Geometry: final body of the model. Coordinates: model frame, mm. Face numbers are marked on the shaded views. A direction names the side the tool comes from. Coordinates: 2 decimals unless noted, no trailing zeros. Loops run counter-clockwise (first coordinate to the right, second up) from the corner with the lowest first, then second, coordinate; pieces in that order, holes last. Notation, with made-up numbers: (-35.5, 42) - (-6.5, 42) arc R11 ccw to (-6.5, 62) - close; hole circle Ø9 at (66, 21). An arc over 180 degrees is marked (long way). Return JSON: item names as keys, results as strings.
from build123d import *

# Parameters (mm, degrees)
SKETCH1_W          = 50.8
SKETCH1_H          = 28.575
EXTRUDE1_DEPTH     = 46.7868
LPATTERN1_COUNT    = 2
LPATTERN1_PITCH    = 27.94
SKETCH5_R          = 13.5001
EXTRUDE2_DEPTH     = 5.969
SKETCH6_W          = 6.3373
SKETCH6_H          = 10.541
CUT_EXTRUDE4_DEPTH = 30.48
HOLE1_D            = 7.137
HOLE1_DEPTH        = 46.7868
HOLE2_D            = 7.137
HOLE2_DEPTH        = 28.575


with BuildPart() as part:
    # Sketch1 → Extrude1 (new body)
    with BuildSketch(Plane(origin=(0, 0, 0), x_dir=(0, 0, -1), z_dir=(1, 0, 0))):
        with Locations((2.3876, 0)):
            Rectangle(SKETCH1_W, SKETCH1_H)
    extrude(amount=EXTRUDE1_DEPTH)

    # S2D0002 → Cut-Revolve1 (revolve, cut)
    with BuildSketch(Plane(origin=(0, 4.7625, 0), x_dir=(-1, 0, 0), z_dir=(0, 1, 0)), mode=Mode.PRIVATE) as cut_revolve1_sk:
        Polygon((-14.5415, -27.5336), (-18.161, -27.5336), (-18.161, -27.7876), (-9.525, -27.7876), (-9.525, -14.0716), (-13.9446, -14.0716), (-13.9446, -26.9113), (-14.5415, -27.5082), align=None)
    cut_revolve1 = revolve(cut_revolve1_sk.sketch.rotate(Axis((9.525, 4.7625, -19.13842003), (0, 0, 1)), 180), axis=Axis((9.525, 4.7625, -19.13842003), (0, 0, 1)), mode=Mode.SUBTRACT)  # turned: the seam where the file's is

    # LPattern1: Cut-Revolve1 ×2
    with Locations(*[(i * LPATTERN1_PITCH, 0, 0) for i in range(1, LPATTERN1_COUNT)]):
        add(cut_revolve1, mode=Mode.SUBTRACT)

    # Sketch5 → Extrude2 (add)
    with BuildSketch(Plane.ZY):
        Circle(SKETCH5_R)
    extrude(amount=EXTRUDE2_DEPTH)

    # Sketch6 → Revolve1 (revolve)
    with BuildSketch(Plane(origin=(0, 0, 0), x_dir=(0, 0, 1), z_dir=(0, -1, 0)), mode=Mode.PRIVATE) as revolve1_sk:
        with Locations((-3.16865, 11.2395)):
            Rectangle(SKETCH6_W, SKETCH6_H)
    revolve(revolve1_sk.sketch.rotate(Axis((5.754582971, 0, 0), (-1, 0, 0)), 180), axis=Axis((5.754582971, 0, 0), (-1, 0, 0)))  # turned: the seam where the file's is

    # S2D0001 → Cut-Revolve4 (revolve, cut)
    with BuildSketch(Plane(origin=(-18.511260017, 3.2639, 0), x_dir=(0, 1, 0), z_dir=(0, 0, 1)), mode=Mode.PRIVATE) as cut_revolve4_sk:
        Polygon((-0.7493, -3.365076823), (-0.7493, -18.003260017), (-3.2639, -19.51418413), (-3.2639, -2.001260017), (0.0381, -2.001260017), align=None)
    revolve(cut_revolve4_sk.sketch.rotate(Axis((0, 0, 0), (-1, 0, 0)), 90), axis=Axis((0, 0, 0), (-1, 0, 0)), mode=Mode.SUBTRACT)  # turned: the seam where the file's is

    # Sketch8 → Cut-Revolve5 (revolve, cut)
    with BuildSketch(Plane(origin=(0, 0, 0), x_dir=(0, 0, -1), z_dir=(0, 1, 0)), mode=Mode.PRIVATE) as cut_revolve5_sk:
        with BuildLine():
            Line((-6.3373, 10.1854), (-6.096, 10.9474))
            Line((-6.096, 10.9474), (-6.096, 15.494))
            ThreePointArc((-6.096, 15.494), (-5.995678675, 16.037796865), (-5.707922533, 16.51))
            Line((-5.707922533, 16.51), (-6.3373, 16.51))
            Line((-6.3373, 16.51), (-6.3373, 10.1854))
        make_face()
    revolve(cut_revolve5_sk.sketch.rotate(Axis((-12.65936, 0, 0), (-1, 0, 0)), 180), axis=Axis((-12.65936, 0, 0), (-1, 0, 0)), mode=Mode.SUBTRACT)  # turned: the seam where the file's is

    # Sketch12 → Cut-Extrude4 (cut, symmetric)
    with BuildSketch(Plane(origin=(0, 0, 0), x_dir=(0, -1, 0), z_dir=(0, 0, -1))):
        Polygon((5.461, 16.51), (5.461, 11.7348), (6.096, 11.0998), (6.096, 16.51), align=None)
        Polygon((-5.461, 16.51), (-5.461, 11.7348), (-6.096, 11.0998), (-6.096, 16.51), align=None)
    extrude(amount=CUT_EXTRUDE4_DEPTH, both=True, mode=Mode.SUBTRACT)

    # Hole1
    with Locations(Plane.ZY):
        with Locations((-16.6878, -7.9248), (16.6624, 7.9502)):
            Hole(HOLE1_D / 2, depth=HOLE1_DEPTH)

    # Hole2
    with Locations(Plane(origin=(0, 14.2875, 0), x_dir=(-1, 0, 0), z_dir=(0, 1, 0))):
        with Locations((-23.3172, -16.6878), (-23.3172, 16.6624)):
            Hole(HOLE2_D / 2, depth=HOLE2_DEPTH)


solid = part.part
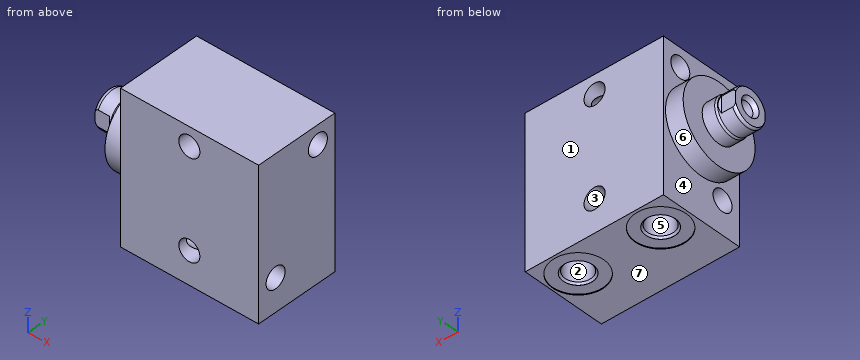
Item 1: Section query C-C, the plane y = -1.75. Count the separate pieces of the cut face and the enclosed holes in it, and give its area (3 significant figures).
Worked out:
{"separate pieces": "1", "enclosed holes": "2", "area": "2,520 mm^2"}
Item 2: Ray query, probe 1 along X at (y, z) = (8, -22.5); probe 2 along Z at (x, y) = (26, 5.5); probe 3 along X at (y, z) = (7.25, 6). Return the intervals inside material, ascending. Write a range as from..to.
Worked out:
{"probe 1": "0..6.52, 12.53..34.46, 40.47..46.79", "probe 2": "-27.79..-19.04, -14.33..14.07, 19.26..23.01", "probe 3": "-5.97..46.79"}
Item 3: Mould query, pull axis X, two halves, no side actions, for the marked faces 1, 2, 3 and 4. Classes: +X half, -X half, draft (parallel to the pull), parting line (faces both ways), or undercut.
Worked out:
{"face 1": "draft", "face 2": "undercut", "face 3": "undercut", "face 4": "-X half"}
Item 4: Reachability of the marked faces 5, 6 and 7 from +Z, -Z, +X, -X, +Y, -Y: full face, straight path, thin tool, end or side. Return the list, or none.
Worked out:
{"face 5": "-Z", "face 6": "-X", "face 7": "-Z, +X, -X, +Y, -Y"}
Item 5: First-contact query: pin 1 Ø11.5 at (y, z) = (7.95, 16.66) entering from -X; pin 2 Ø4 at (x, z) = (-14.5, -1) entering from -Y; pin 3 Ø8 at (x, y) = (37.47, 4.76) entering from -Z. Flat tips, straight axial feed; report the tip coordinate or a pass-through.
Worked out:
{"pin 1": "x = -5.97", "pin 2": "y = -5.46", "pin 3": "z = -14.07"}
Item 6: Section query A-A, the plane z = -19. Return loops of the section in (x, y) (1 decimal).
Worked out:
{"outline": "(0, -14.3) - (20.6, -14.3) - (20.6, -10.6) - (0, -10.6) - close; (0, -5.2) - (20.6, -5.2) - (20.6, 14.3) - (0, 14.3) - close; (26, -14.3) - (46.8, -14.3) - (46.8, -10.6) - (26, -10.6) - close; (26, -5.2) - (46.8, -5.2) - (46.8, 14.3) - (26, 14.3) - close; hole circle Ø8.8 at (9.5, 4.8); hole circle Ø8.8 at (37.5, 4.8)"}
Item 7: Section query B-B, the plane z = 17.5. Return loops of the section in (x, y), and give its area (3 significant figures).
Worked out:
{"outline": "(0, -14.29) - (19.85, -14.29) - (19.85, 4.48) - (0, 4.48) - close; (0, 11.42) - (19.85, 11.42) - (19.85, 14.29) - (0, 14.29) - close; (26.79, -14.29) - (46.79, -14.29) - (46.79, 4.48) - (26.79, 4.48) - close; (26.79, 11.42) - (46.79, 11.42) - (46.79, 14.29) - (26.79, 14.29) - close", "area": "862 mm^2"}
